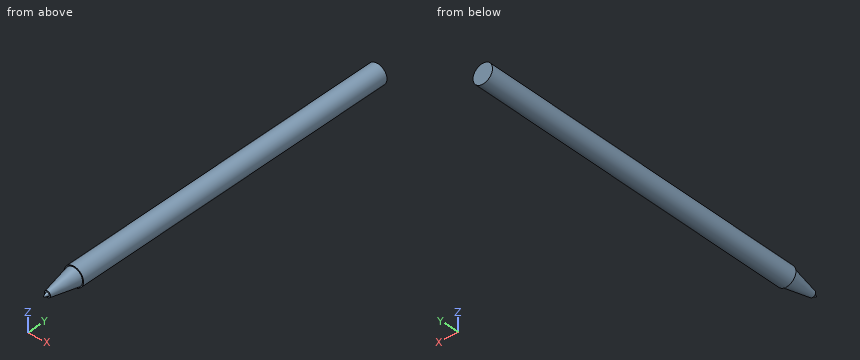
from build123d import *

# Parameters (mm, degrees)
SKETCH1_R           = 4
BOSS_EXTRUDE1_DEPTH = 138
SKETCH2_R           = 3.6
BOSS_EXTRUDE2_DEPTH = 12
BOSS_EXTRUDE2_TAPER = 11


with BuildPart() as part:
    # Sketch1 → Boss-Extrude1 (new body)
    with BuildSketch(Plane(origin=(0, 0, 0), x_dir=(1, 0, 0), z_dir=(0, 1, 0))):
        with Locations(Location((0, 0, 0), (0, 0, 270))):
            Circle(SKETCH1_R)
    extrude(amount=BOSS_EXTRUDE1_DEPTH)

    # Sketch2 → Boss-Extrude2 (add)
    with BuildSketch(Plane.XZ):
        Circle(SKETCH2_R)
    extrude(amount=BOSS_EXTRUDE2_DEPTH, taper=BOSS_EXTRUDE2_TAPER)

    # Boss-Extrude3 cone 1 section (through the dimple's axis) → Boss-Extrude3 (revolve)
    with BuildSketch(Plane(origin=(0, -12, 0), x_dir=(0, 0, 1), z_dir=(1, 0, 0))):
        Polygon((0, 0), (0.76743629, 0), (0, 1.999239888), align=None)
    revolve(axis=Axis((0, -12, 0), (0, -1, 0)))


solid = part.part
CAD build for the part. Positions are in the model's coordinates, mm. Round coordinates to 2 decimals unless told otherwise and drop trailing zeros. Loops run counter-clockwise (first coordinate to the right, second up) from the corner with the lowest first, then second, coordinate; pieces in that order, holes last. Notation, with made-up numbers: (-11.75, 40.5) - (5.25, 40.5) arc R14 ccw to (5.25, 61.5) - close; hole circle Ø3 at (73, 62). An arc over 180 degrees is marked (long way). Put each result on its own line as item: value.
1. Wall check: line 1 (X direction, y = 13, z = 0.25); line 2 (Y direction, x = 3, z = -2.5); line 3 (Y direction, x = 0, z = -1). Give the ranges that are in metal, low to high.
Geometry check:
line 1: -3.99 to 3.99
line 2: 0 to 138
line 3: -12 to 138
2. Pin check, flat tips, straight feed: P1, Ø2, axis at x = -0.5, y = 31.5, coming from the +Z side; P2, Ø3, axis at y = 88.5, z = 2, coming from the +X side. Stop position of each tip, or through.
Geometry check:
P1: z = 4
P2: x = 3.97
3. Slice it at A-A on y = 49. List the corners of the cut face in (x, z).
Geometry check:
outline: circle Ø8 at (0, 0)
